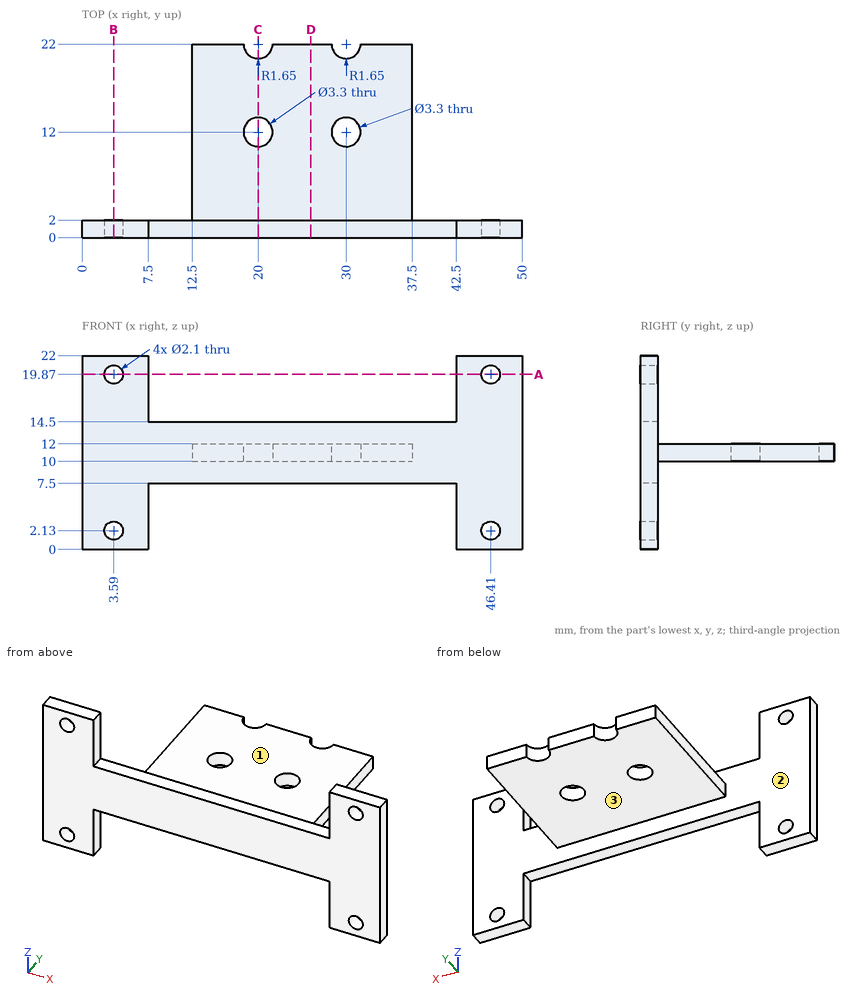
Part print with two shaded views. Sizes in mm from the minimum x, y, z corner. Round coordinates to 2 decimals unless told otherwise and drop trailing zeros. Loops run counter-clockwise (first coordinate to the right, second up) from the corner with the lowest first, then second, coordinate; pieces in that order, holes last. Notation, with made-up numbers: (31, 14.25) - (40, 14.25) arc R13 cw to (40, 35.25) - close; hole circle Ø1 at (42, 75). An arc over 180 degrees is marked (long way). Put each result on its own line as item: value.
1. Slice it at B-B on x = 3.59. List the corners of the cut face in (y, z), and give its area (3 significant figures).
Geometry check:
outline: (0, 0) - (2, 0) - (2, 1.08) - (0, 1.08) - close; (0, 3.18) - (2, 3.18) - (2, 18.82) - (0, 18.82) - close; (0, 20.92) - (2, 20.92) - (2, 22) - (0, 22) - close
area: 35.6 mm²
2. Slice it at C-C on x = 20. List the corners of the cut face in (y, z).
Geometry check:
outline: (0, 7.5) - (2, 7.5) - (2, 10) - (10.35, 10) - (10.35, 12) - (2, 12) - (2, 14.5) - (0, 14.5) - close; (13.65, 10) - (20.35, 10) - (20.35, 12) - (13.65, 12) - close
3. Wall check: line 1 (X direction, y = 0.65, z = 19.87); line 2 (Y direction, x = 2, z = 14.25); line 3 (Z direction, x = 18, y = 13.5). Give the ranges that are in metal, low to high.
Geometry check:
line 1: 0 to 2.54, 4.64 to 7.5, 42.5 to 45.36, 47.46 to 50
line 2: 0 to 2
line 3: 10 to 12
4. Two-plate mould, pull along Z, no slides. Class the marked faces 1, 2 and 3: released by +Z, released by -Z, zero draft, split by the parting line, or undercut.
Geometry check:
face 1: released by +Z
face 2: zero draft
face 3: released by -Z
5. Slice it at D-D on x = 26. List the corners of the cut face in (y, z).
Geometry check:
outline: (0, 7.5) - (2, 7.5) - (2, 10) - (22, 10) - (22, 12) - (2, 12) - (2, 14.5) - (0, 14.5) - close
6. Pin check, flat tips, straight feed: P1, Ø4, axis at x = 20, y = 12, coming from the +Z side; P2, Ø8, axis at x = 26, z = 4, coming from the +Y side; P3, Ø10, axis at x = 25.5, y = 4.5, coming from the -Z side; P4, Ø4, axis at y = 15.5, z = 6.5, coming from the +X side. Stop position of each tip, or through.
Geometry check:
P1: z = 12
P2: y = 2
P3: z = 7.5
P4: through
7. Slice it at A-A on z = 19.87. List the corners of the cut face in (x, y).
Geometry check:
outline: (0, 0) - (2.54, 0) - (2.54, 2) - (0, 2) - close; (4.64, 0) - (7.5, 0) - (7.5, 2) - (4.64, 2) - close; (42.5, 0) - (45.36, 0) - (45.36, 2) - (42.5, 2) - close; (47.46, 0) - (50, 0) - (50, 2) - (47.46, 2) - close
